```python
from build123d import *

# Parameters (mm, degrees)
BOSS_EXTRUDE1_DEPTH      = 3.81
BOSS_EXTRUDE1_DEPTH_BACK = 3.81
SKETCH3_W                = 2.783274099
SKETCH3_H                = 5.656099036
BOSS_EXTRUDE2_DEPTH      = 7.62


with BuildPart() as part:
    # Sketch2 → Boss-Extrude1 (new, two sides: drawn at the far end of the back side and taken through both)
    with BuildSketch(Plane(origin=(-2.32915921, 0, 0), x_dir=(0, 0, -1), z_dir=(1, 0, 0)).offset(-BOSS_EXTRUDE1_DEPTH_BACK)):
        with BuildLine():
            Line((-11.339007657, 18.600950631), (-11.339007657, 8.436760495))
            Line((-11.339007657, 8.436760495), (-7.601027883, -0.203787431))
            Line((-7.601027883, -0.203787431), (6.154737684, -0.203787431))
            Line((6.154737684, -0.203787431), (9.668438671, 7.945008476))
            Line((9.668438671, 7.945008476), (9.668438671, 18.600950631))
            ThreePointArc((9.668438671, 18.600950631), (-0.835284493, 25.430388096), (-11.339007657, 18.600950631))
        make_face()
        with BuildLine():
            Line((8.923024063, 18.600950631), (8.923024063, 8.436760495))
            Line((8.923024063, 8.436760495), (5.557346164, 0.521588901))
            Line((5.557346164, 0.521588901), (-7.142653836, 0.521588901))
            Line((-7.142653836, 0.521588901), (-10.584175937, 8.436760495))
            Line((-10.584175937, 8.436760495), (-10.584175937, 18.600950631))
            ThreePointArc((-10.584175937, 18.600950631), (-0.830575937, 24.692849221), (8.923024063, 18.600950631))
        make_face(mode=Mode.SUBTRACT)
    extrude(amount=BOSS_EXTRUDE1_DEPTH + BOSS_EXTRUDE1_DEPTH_BACK)

    # Sketch3 → Boss-Extrude2 (add)
    with BuildSketch(Plane(origin=(1.48084079, 0, 0), x_dir=(0, 0, -1), z_dir=(1, 0, 0))):
        with Locations((-12.730644707, 11.264810013)):
            Rectangle(SKETCH3_W, SKETCH3_H)
    extrude(amount=-BOSS_EXTRUDE2_DEPTH)


solid = part.part
```
The model under review builds one solid part; all positions refer to its coordinate system, in mm. A direction names the side the tool comes from. Coordinates: 2 decimals unless noted, no trailing zeros. Write each loop counter-clockwise with the first axis right and the second up, starting at its lowest first coordinate (ties: lowest second). Pieces come first, ordered by that corner, then holes. Notation, with made-up numbers: (-27, 83.25) - (17, 83.25) arc R31 ccw to (17, 110.25) - close; hole circle Ø2 at (32, -36.5). An arc over 180 degrees is marked (long way). Answer in a Markdown table with one row per item. Add a question column.
Q1. For faces 1 (the face through (-2, 16, 11.339)), 2 (the face through (-2, 13, -9.668)), 3 (the face through (-2, 14, -8.923)), 4 (the face through (-2, 8.437, 13)), list the 3-axis set-ups (+Z, -Z, +X, -X, +Y, -Y) from which the entire face can be reached by the end or side of a thin tool; tool diameter is ignored.
Q2. Consider section A-A on y = 9. Give the boundary of the cut face in (x, z).
Q3. Draft analysis for pull direction Y (two halves, no side actions). For faces 5 (the face through (-2.382, 4.424, 8.839)), 6 (the face through (-2, 14.093, 13)), 7 (the face through (-2, 11, 14.122)), state which applies: +Y half, -Y half, draft (parallel to the pull), parting line (faces both ways), or undercut.
Q4. To check wall thickness, follow line 1 along Z through (x, y) = (-4.75, 12); line 2 along Z through (x, y) = (-1.25, 16.5); line 3 along Y through (x, z) = (-3.5, 2). State the ranges of each line that lie inside material, in increasing order. Write a range as from..to.
Q5. Clearance check with flat-ended pins moving along their axes: pin 1 (3 mm diameter, centred on x = -4, z = 13, fed in from +Y); pin 2 (1 mm diameter, centred on y = 20, z = -6, fed in from -X); pin 3 (2 mm diameter, centred on x = -2.5, z = 13.5, fed in from -Y); pin 4 (3.5 mm diameter, centred on x = -2.5, y = 17, fed in from +Z). State where each tip first meets the part, or that it passes through.
Q6. Consider section B-B on z = 6.25. Give the boundary of the cut face in (x, y), then the cut area to 3 significant figures.
Q7. Consider section C-C on x = -3.75. Give the boundary of the cut face in (y, z) (3 decimals).
Answers below:
| question | item | result |
|---|---|---|
| 1 | face 1 | +Z, +X, -X, +Y |
| 1 | face 2 | -Z, +X, -X, +Y, -Y |
| 1 | face 3 | +X, -X |
| 1 | face 4 | +Z, +X, -X, -Y |
| 2 | outline | (-6.14, -9.67) - (1.48, -9.67) - (1.48, -8.92) - (-6.14, -8.92) - close; (-6.14, 10.58) - (1.48, 10.58) - (1.48, 14.12) - (-6.14, 14.12) - close |
| 3 | face 5 | undercut |
| 3 | face 6 | +Y half |
| 3 | face 7 | draft |
| 4 | line 1 | -9.67..-8.92, 10.58..14.12 |
| 4 | line 2 | -9.67..-8.92, 10.58..11.34 |
| 4 | line 3 | -0.2..0.52, 24.63..25.37 |
| 5 | pin 1 | y = 14.09 |
| 5 | pin 2 | through |
| 5 | pin 3 | y = 8.44 |
| 5 | pin 4 | z = 11.34 |
| 6 | outline | (-6.14, -0.2) - (1.48, -0.2) - (1.48, 0.52) - (-6.14, 0.52) - close; (-6.14, 23.24) - (1.48, 23.24) - (1.48, 24.07) - (-6.14, 24.07) - close |
| 6 | area | 11.9 mm² |
| 7 | outline | (-0.204, -6.155) - (7.945, -9.668) - (18.601, -9.668) arc R11.492 ccw to (18.601, 11.339) - (14.093, 11.339) - (14.093, 14.122) - (8.437, 14.122) - (8.437, 11.339) - (-0.204, 7.601) - close; hole (0.522, -5.557) - (8.437, -8.923) - (18.601, -8.923) arc R10.854 ccw to (18.601, 10.584) - (8.437, 10.584) - (0.522, 7.143) - close |
